For this review, take the finished solid that the model builds, in its own axes (mm). A direction names the side the tool comes from. Coordinates: 2 decimals unless noted, no trailing zeros. Loops run counter-clockwise (first coordinate to the right, second up) from the corner with the lowest first, then second, coordinate; pieces in that order, holes last. Notation, with made-up numbers: M 79,55.25 L 87,55.25 A7 cw 87,61.25 Z; hole C -26,60 d6. An arc over 180 degrees is marked long. Write item = value, one per line.
from build123d import *

# Parameters (mm, degrees)
SKETCH_1_R      = 1.5
EXTRUDE_1_DEPTH = 4
CHAMFER_1_SIZE  = 0.1


with BuildPart() as part:
    # 草图1 → 凸台-拉伸1 (new body)
    with BuildSketch(Plane(origin=(4, 0, 0), x_dir=(0, 0, -1), z_dir=(1, 0, 0))):
        with BuildLine():
            ThreePointArc((-5.368564348, 0.241646108), (-5.374, 0), (-5.368564348, -0.241646108))
            ThreePointArc((-5.368564348, -0.241646108), (-5.94431135, -0.407766737), (-6.460959589, -0.711337602))
            ThreePointArc((-6.460959589, -0.711337602), (-6.444391599, -0.848420249), (-6.424915449, -0.98512003))
            ThreePointArc((-6.424915449, -0.98512003), (-5.84730165, -1.144628565), (-5.248177569, -1.156074481))
            ThreePointArc((-5.248177569, -1.156074481), (-5.19088539, -1.390893548), (-5.123092339, -1.622898915))
            ThreePointArc((-5.123092339, -1.622898915), (-5.636226055, -1.93237341), (-6.056700011, -2.359318752))
            ThreePointArc((-6.056700011, -2.359318752), (-6.005216961, -2.48744231), (-5.951023938, -2.614443361))
            ThreePointArc((-5.951023938, -2.614443361), (-5.351808006, -2.619019322), (-4.770136161, -2.475010506))
            ThreePointArc((-4.770136161, -2.475010506), (-4.65402052, -2.687), (-4.528490053, -2.893553842))
            ThreePointArc((-4.528490053, -2.893553842), (-4.944041268, -3.325292028), (-5.239686336, -3.846516229))
            ThreePointArc((-5.239686336, -3.846516229), (-5.156796712, -3.956949289), (-5.071579981, -4.065596697))
            ThreePointArc((-5.071579981, -4.065596697), (-4.49159749, -3.91492824), (-3.967017857, -3.625278654))
            ThreePointArc((-3.967017857, -3.625278654), (-3.799991842, -3.799991842), (-3.625278654, -3.967017857))
            ThreePointArc((-3.625278654, -3.967017857), (-3.91492824, -4.49159749), (-4.065596697, -5.071579981))
            ThreePointArc((-4.065596697, -5.071579981), (-3.956949289, -5.156796712), (-3.846516229, -5.239686336))
            ThreePointArc((-3.846516229, -5.239686336), (-3.325292028, -4.944041268), (-2.893553842, -4.528490053))
            ThreePointArc((-2.893553842, -4.528490053), (-2.687, -4.65402052), (-2.475010506, -4.770136161))
            ThreePointArc((-2.475010506, -4.770136161), (-2.619019322, -5.351808006), (-2.614443361, -5.951023938))
            ThreePointArc((-2.614443361, -5.951023938), (-2.48744231, -6.005216961), (-2.359318752, -6.056700011))
            ThreePointArc((-2.359318752, -6.056700011), (-1.93237341, -5.636226055), (-1.622898915, -5.123092339))
            ThreePointArc((-1.622898915, -5.123092339), (-1.390893548, -5.19088539), (-1.156074481, -5.248177569))
            ThreePointArc((-1.156074481, -5.248177569), (-1.144628565, -5.84730165), (-0.98512003, -6.424915449))
            ThreePointArc((-0.98512003, -6.424915449), (-0.848420249, -6.444391599), (-0.711337602, -6.460959589))
            ThreePointArc((-0.711337602, -6.460959589), (-0.407766737, -5.94431135), (-0.241646108, -5.368564348))
            ThreePointArc((-0.241646108, -5.368564348), (0, -5.374), (0.241646108, -5.368564348))
            ThreePointArc((0.241646108, -5.368564348), (0.407766737, -5.94431135), (0.711337602, -6.460959589))
            ThreePointArc((0.711337602, -6.460959589), (0.848420249, -6.444391599), (0.98512003, -6.424915449))
            ThreePointArc((0.98512003, -6.424915449), (1.144628565, -5.84730165), (1.156074481, -5.248177569))
            ThreePointArc((1.156074481, -5.248177569), (1.390893548, -5.19088539), (1.622898915, -5.123092339))
            ThreePointArc((1.622898915, -5.123092339), (1.93237341, -5.636226055), (2.359318752, -6.056700011))
            ThreePointArc((2.359318752, -6.056700011), (2.48744231, -6.005216961), (2.614443361, -5.951023938))
            ThreePointArc((2.614443361, -5.951023938), (2.619019322, -5.351808006), (2.475010506, -4.770136161))
            ThreePointArc((2.475010506, -4.770136161), (2.687, -4.65402052), (2.893553842, -4.528490053))
            ThreePointArc((2.893553842, -4.528490053), (3.325292028, -4.944041268), (3.846516229, -5.239686336))
            ThreePointArc((3.846516229, -5.239686336), (3.956949289, -5.156796712), (4.065596697, -5.071579981))
            ThreePointArc((4.065596697, -5.071579981), (3.91492824, -4.49159749), (3.625278654, -3.967017857))
            ThreePointArc((3.625278654, -3.967017857), (3.799991842, -3.799991842), (3.967017857, -3.625278654))
            ThreePointArc((3.967017857, -3.625278654), (4.49159749, -3.91492824), (5.071579981, -4.065596697))
            ThreePointArc((5.071579981, -4.065596697), (5.156796712, -3.956949289), (5.239686336, -3.846516229))
            ThreePointArc((5.239686336, -3.846516229), (4.944041268, -3.325292028), (4.528490053, -2.893553842))
            ThreePointArc((4.528490053, -2.893553842), (4.65402052, -2.687), (4.770136161, -2.475010506))
            ThreePointArc((4.770136161, -2.475010506), (5.351808006, -2.619019322), (5.951023938, -2.614443361))
            ThreePointArc((5.951023938, -2.614443361), (6.005216961, -2.48744231), (6.056700011, -2.359318752))
            ThreePointArc((6.056700011, -2.359318752), (5.636226055, -1.93237341), (5.123092339, -1.622898915))
            ThreePointArc((5.123092339, -1.622898915), (5.19088539, -1.390893548), (5.248177569, -1.156074481))
            ThreePointArc((5.248177569, -1.156074481), (5.84730165, -1.144628565), (6.424915449, -0.98512003))
            ThreePointArc((6.424915449, -0.98512003), (6.444391599, -0.848420249), (6.460959589, -0.711337602))
            ThreePointArc((6.460959589, -0.711337602), (5.94431135, -0.407766737), (5.368564348, -0.241646108))
            ThreePointArc((5.368564348, -0.241646108), (5.374, 0), (5.368564348, 0.241646108))
            ThreePointArc((5.368564348, 0.241646108), (5.94431135, 0.407766737), (6.460959589, 0.711337602))
            ThreePointArc((6.460959589, 0.711337602), (6.444391599, 0.848420249), (6.424915449, 0.98512003))
            ThreePointArc((6.424915449, 0.98512003), (5.84730165, 1.144628565), (5.248177569, 1.156074481))
            ThreePointArc((5.248177569, 1.156074481), (5.19088539, 1.390893548), (5.123092339, 1.622898915))
            ThreePointArc((5.123092339, 1.622898915), (5.636226055, 1.93237341), (6.056700011, 2.359318752))
            ThreePointArc((6.056700011, 2.359318752), (6.005216961, 2.48744231), (5.951023938, 2.614443361))
            ThreePointArc((5.951023938, 2.614443361), (5.351808006, 2.619019322), (4.770136161, 2.475010506))
            ThreePointArc((4.770136161, 2.475010506), (4.65402052, 2.687), (4.528490053, 2.893553842))
            ThreePointArc((4.528490053, 2.893553842), (4.944041268, 3.325292028), (5.239686336, 3.846516229))
            ThreePointArc((5.239686336, 3.846516229), (5.156796712, 3.956949289), (5.071579981, 4.065596697))
            ThreePointArc((5.071579981, 4.065596697), (4.49159749, 3.91492824), (3.967017857, 3.625278654))
            ThreePointArc((3.967017857, 3.625278654), (3.799991842, 3.799991842), (3.625278654, 3.967017857))
            ThreePointArc((3.625278654, 3.967017857), (3.91492824, 4.49159749), (4.065596697, 5.071579981))
            ThreePointArc((4.065596697, 5.071579981), (3.956949289, 5.156796712), (3.846516229, 5.239686336))
            ThreePointArc((3.846516229, 5.239686336), (3.325292028, 4.944041268), (2.893553842, 4.528490053))
            ThreePointArc((2.893553842, 4.528490053), (2.687, 4.65402052), (2.475010506, 4.770136161))
            ThreePointArc((2.475010506, 4.770136161), (2.619019322, 5.351808006), (2.614443361, 5.951023938))
            ThreePointArc((2.614443361, 5.951023938), (2.48744231, 6.005216961), (2.359318752, 6.056700011))
            ThreePointArc((2.359318752, 6.056700011), (1.93237341, 5.636226055), (1.622898915, 5.123092339))
            ThreePointArc((1.622898915, 5.123092339), (1.390893548, 5.19088539), (1.156074481, 5.248177569))
            ThreePointArc((1.156074481, 5.248177569), (1.144628565, 5.84730165), (0.98512003, 6.424915449))
            ThreePointArc((0.98512003, 6.424915449), (0.848420249, 6.444391599), (0.711337602, 6.460959589))
            ThreePointArc((0.711337602, 6.460959589), (0.407766737, 5.94431135), (0.241646108, 5.368564348))
            ThreePointArc((0.241646108, 5.368564348), (0, 5.374), (-0.241646108, 5.368564348))
            ThreePointArc((-0.241646108, 5.368564348), (-0.407766737, 5.94431135), (-0.711337602, 6.460959589))
            ThreePointArc((-0.711337602, 6.460959589), (-0.848420249, 6.444391599), (-0.98512003, 6.424915449))
            ThreePointArc((-0.98512003, 6.424915449), (-1.144628565, 5.84730165), (-1.156074481, 5.248177569))
            ThreePointArc((-1.156074481, 5.248177569), (-1.390893548, 5.19088539), (-1.622898915, 5.123092339))
            ThreePointArc((-1.622898915, 5.123092339), (-1.93237341, 5.636226055), (-2.359318752, 6.056700011))
            ThreePointArc((-2.359318752, 6.056700011), (-2.48744231, 6.005216961), (-2.614443361, 5.951023938))
            ThreePointArc((-2.614443361, 5.951023938), (-2.619019322, 5.351808006), (-2.475010506, 4.770136161))
            ThreePointArc((-2.475010506, 4.770136161), (-2.687, 4.65402052), (-2.893553842, 4.528490053))
            ThreePointArc((-2.893553842, 4.528490053), (-3.325292028, 4.944041268), (-3.846516229, 5.239686336))
            ThreePointArc((-3.846516229, 5.239686336), (-3.956949289, 5.156796712), (-4.065596697, 5.071579981))
            ThreePointArc((-4.065596697, 5.071579981), (-3.91492824, 4.49159749), (-3.625278654, 3.967017857))
            ThreePointArc((-3.625278654, 3.967017857), (-3.799991842, 3.799991842), (-3.967017857, 3.625278654))
            ThreePointArc((-3.967017857, 3.625278654), (-4.49159749, 3.91492824), (-5.071579981, 4.065596697))
            ThreePointArc((-5.071579981, 4.065596697), (-5.156796712, 3.956949289), (-5.239686336, 3.846516229))
            ThreePointArc((-5.239686336, 3.846516229), (-4.944041268, 3.325292028), (-4.528490053, 2.893553842))
            ThreePointArc((-4.528490053, 2.893553842), (-4.65402052, 2.687), (-4.770136161, 2.475010506))
            ThreePointArc((-4.770136161, 2.475010506), (-5.351808006, 2.619019322), (-5.951023938, 2.614443361))
            ThreePointArc((-5.951023938, 2.614443361), (-6.005216961, 2.48744231), (-6.056700011, 2.359318752))
            ThreePointArc((-6.056700011, 2.359318752), (-5.636226055, 1.93237341), (-5.123092339, 1.622898915))
            ThreePointArc((-5.123092339, 1.622898915), (-5.19088539, 1.390893548), (-5.248177569, 1.156074481))
            ThreePointArc((-5.248177569, 1.156074481), (-5.84730165, 1.144628565), (-6.424915449, 0.98512003))
            ThreePointArc((-6.424915449, 0.98512003), (-6.444391599, 0.848420249), (-6.460959589, 0.711337602))
            ThreePointArc((-6.460959589, 0.711337602), (-5.94431135, 0.407766737), (-5.368564348, 0.241646108))
        make_face()
        with Locations(Location((0, 0, 0), (0, 0, 180))):
            Circle(SKETCH_1_R, mode=Mode.SUBTRACT)
    extrude(amount=-EXTRUDE_1_DEPTH)

    # 倒角1
    chamfer_1_edges = [part.edges().sort_by_distance(p)[0] for p in [
        (0, 0, -1.5),
    ]]
    chamfer(chamfer_1_edges, length=CHAMFER_1_SIZE)


solid = part.part
Q1. Add section D-D (z = 2). Write out the cut boundary in (x, y), and give its area (3 significant figures).
Solved:
outline = M 0,-5.72 L 4,-5.72 L 4,5.72 L 0,5.72 Z
area = 45.7 mm²
Q2. Draft analysis for pull direction Y (two halves, no side actions). For faces 1 (the face through (0, 2, 2)), 2 (the face through (2.03, 5.63, 1.93)), 3 (the face through (2.03, 3.32, -4.94)), 4 (the face through (2.03, -1.93, 5.63)), state which applies: +Y half, -Y half, draft (parallel to the pull), parting line (faces both ways), or undercut.
Solved:
face_1 = draft
face_2 = +Y half
face_3 = undercut
face_4 = undercut
Q3. Add section C-C (y = 5.75). Write out the cut boundary in (x, z).
Solved:
outline = M 0,-2.63 L 4,-2.63 L 4,-2.03 L 0,-2.03 Z; M 0,-1.16 L 4,-1.16 L 4,-0.33 L 0,-0.33 Z; M 0,0.33 L 4,0.33 L 4,1.16 L 0,1.16 Z; M 0,2.03 L 4,2.03 L 4,2.63 L 0,2.63 Z
Q4. For pin 1 Ø3.5 at (y, z) = (0, 0) entering from +X; pin 2 Ø1 at (x, z) = (0.5, -2) entering from +Y; pin 3 Ø2 at (x, z) = (2.5, -3.5) entering from +Y, all flat-tipped, find the tip position at first contact; note any pin that passes through.
Solved:
pin_1 = 4
pin_2 = 6.06
pin_3 = 6
Q5. Add section A-A (z = 0). Write out the cut boundary in (x, y), and give its area (3 significant figures).
Solved:
outline = M 0,-5.37 L 4,-5.37 L 4,-1.5 L 0.1,-1.5 L 0,-1.6 Z; M 0,1.6 L 0.1,1.5 L 4,1.5 L 4,5.37 L 0,5.37 Z
area = 31.0 mm²
Q6. For line 1 along Y through (x, z) = (2.1, -5.5); line 2 along Y through (x, z) = (0.95, 0); line 3 along Z through (x, y) = (2.4, 1.25), list the stretches that pass through material, from the lowest coordinate up.
Solved:
line_1 = -2.63 to -1.83, -1.17 to -0.27, 0.27 to 1.17, 1.83 to 2.63
line_2 = -5.37 to -1.5, 1.5 to 5.37
line_3 = -5.23 to -0.83, 0.83 to 5.23
Q7. Machinability: for faces 5 (the face through (2.028, 1.938, 5.643)), 6 (the face through (2.03, -5.63, -1.93)), 7 (the face through (2.03, 4.95, -3.33)), 8 (the face through (2.028, 5.839, -1.146)), 9 (the face through (2.03, 1.93, -5.63)), which of the approach directions +Z, -Z, +X, -X, +Y, -Y give a long, thin tool a straight path to every point of the face, cutting with its end or side? Answer none if there is none.
Solved:
face_5 = +Z, +X, -X
face_6 = +X, -X, -Y
face_7 = +X, -X, +Y
face_8 = +X, -X
face_9 = -Z, +X, -X
